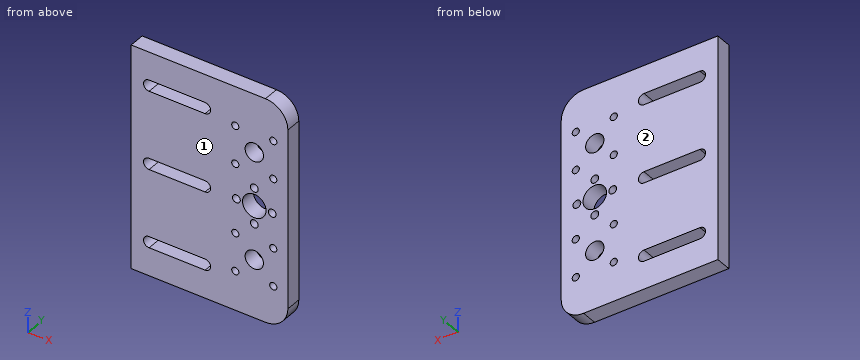
from build123d import *

# Parameters (mm, degrees)
SKETCH1_R           = 1.6
SKETCH1_R_2         = 4.1
SKETCH1_R_3         = 1.75
SKETCH1_R_4         = 5.25
BOSS_EXTRUDE1_DEPTH = 7
FILLET1_R           = 10


with BuildPart() as part:
    # Sketch1 → Boss-Extrude1 (new body)
    # profile 1 of 3: a face of its own
    with BuildSketch(Plane(origin=(0, 0, 0), x_dir=(1, 0, 0), z_dir=(0, 1, 0))):
        Polygon((0, 100), (0, 0), (56, 0), (70, 0), (70, 100), align=None)
        with BuildLine():
            Line((33, 12.5), (8, 12.5))
            ThreePointArc((8, 12.5), (5.5, 15), (8, 17.5))
            Line((8, 17.5), (33, 17.5))
            ThreePointArc((33, 17.5), (35.5, 15), (33, 12.5))
        make_face(mode=Mode.SUBTRACT)
        with Locations(Location((46.51, 17.51, 0), (0, 0, 270))):
            Circle(SKETCH1_R, mode=Mode.SUBTRACT)
        with Locations(Location((63.49, 17.51, 0), (0, 0, 270))):
            Circle(SKETCH1_R, mode=Mode.SUBTRACT)
        with Locations(Location((46.51, 34.49, 0), (0, 0, 270))):
            Circle(SKETCH1_R, mode=Mode.SUBTRACT)
        with Locations(Location((55, 26, 0), (0, 0, 270))):
            Circle(SKETCH1_R_2, mode=Mode.SUBTRACT)
        with Locations(Location((63.49, 34.49, 0), (0, 0, 270))):
            Circle(SKETCH1_R, mode=Mode.SUBTRACT)
        with Locations(Location((55, 42, 0), (0, 0, 270))):
            Circle(SKETCH1_R_3, mode=Mode.SUBTRACT)
        with BuildLine():
            ThreePointArc((8, 47.5), (5.5, 50), (8, 52.5))
            Line((8, 52.5), (33, 52.5))
            ThreePointArc((33, 52.5), (35.5, 50), (33, 47.5))
            Line((33, 47.5), (8, 47.5))
        make_face(mode=Mode.SUBTRACT)
        with BuildLine():
            ThreePointArc((8, 82.5), (5.5, 85), (8, 87.5))
            Line((8, 87.5), (33, 87.5))
            ThreePointArc((33, 87.5), (35.5, 85), (33, 82.5))
            Line((33, 82.5), (8, 82.5))
        make_face(mode=Mode.SUBTRACT)
        with Locations(Location((47, 50, 0), (0, 0, 270))):
            Circle(SKETCH1_R_3, mode=Mode.SUBTRACT)
        with Locations(Location((46.51, 65.51, 0), (0, 0, 270))):
            Circle(SKETCH1_R, mode=Mode.SUBTRACT)
        with Locations(Location((55, 50, 0), (0, 0, 270))):
            Circle(SKETCH1_R_4, mode=Mode.SUBTRACT)
        with Locations(Location((55, 58, 0), (0, 0, 270))):
            Circle(SKETCH1_R_3, mode=Mode.SUBTRACT)
        with Locations(Location((63, 50, 0), (0, 0, 270))):
            Circle(SKETCH1_R_3, mode=Mode.SUBTRACT)
        with Locations(Location((55, 74, 0), (0, 0, 270))):
            Circle(SKETCH1_R_2, mode=Mode.SUBTRACT)
        with Locations(Location((63.49, 65.51, 0), (0, 0, 270))):
            Circle(SKETCH1_R, mode=Mode.SUBTRACT)
        with Locations(Location((46.51, 82.49, 0), (0, 0, 270))):
            Circle(SKETCH1_R, mode=Mode.SUBTRACT)
        with Locations(Location((63.49, 82.49, 0), (0, 0, 270))):
            Circle(SKETCH1_R, mode=Mode.SUBTRACT)
    # profile 2 of 3: a face of its own
    with BuildSketch(Plane(origin=(0, 0, 0), x_dir=(1, 0, 0), z_dir=(0, 1, 0))):
        Polygon((0, 100), (0, 0), (56, 0), (70, 0), (70, 100), align=None)
        with BuildLine():
            Line((33, 12.5), (8, 12.5))
            ThreePointArc((8, 12.5), (5.5, 15), (8, 17.5))
            Line((8, 17.5), (33, 17.5))
            ThreePointArc((33, 17.5), (35.5, 15), (33, 12.5))
        make_face(mode=Mode.SUBTRACT)
        with Locations(Location((46.51, 17.51, 0), (0, 0, 270))):
            Circle(SKETCH1_R, mode=Mode.SUBTRACT)
        with Locations(Location((63.49, 17.51, 0), (0, 0, 270))):
            Circle(SKETCH1_R, mode=Mode.SUBTRACT)
        with Locations(Location((46.51, 34.49, 0), (0, 0, 270))):
            Circle(SKETCH1_R, mode=Mode.SUBTRACT)
        with Locations(Location((55, 26, 0), (0, 0, 270))):
            Circle(SKETCH1_R_2, mode=Mode.SUBTRACT)
        with Locations(Location((63.49, 34.49, 0), (0, 0, 270))):
            Circle(SKETCH1_R, mode=Mode.SUBTRACT)
        with Locations(Location((55, 42, 0), (0, 0, 270))):
            Circle(SKETCH1_R_3, mode=Mode.SUBTRACT)
        with BuildLine():
            ThreePointArc((8, 47.5), (5.5, 50), (8, 52.5))
            Line((8, 52.5), (33, 52.5))
            ThreePointArc((33, 52.5), (35.5, 50), (33, 47.5))
            Line((33, 47.5), (8, 47.5))
        make_face(mode=Mode.SUBTRACT)
        with BuildLine():
            ThreePointArc((8, 82.5), (5.5, 85), (8, 87.5))
            Line((8, 87.5), (33, 87.5))
            ThreePointArc((33, 87.5), (35.5, 85), (33, 82.5))
            Line((33, 82.5), (8, 82.5))
        make_face(mode=Mode.SUBTRACT)
        with Locations(Location((47, 50, 0), (0, 0, 270))):
            Circle(SKETCH1_R_3, mode=Mode.SUBTRACT)
        with Locations(Location((46.51, 65.51, 0), (0, 0, 270))):
            Circle(SKETCH1_R, mode=Mode.SUBTRACT)
        with Locations(Location((55, 50, 0), (0, 0, 270))):
            Circle(SKETCH1_R_4, mode=Mode.SUBTRACT)
        with Locations(Location((55, 58, 0), (0, 0, 270))):
            Circle(SKETCH1_R_3, mode=Mode.SUBTRACT)
        with Locations(Location((63, 50, 0), (0, 0, 270))):
            Circle(SKETCH1_R_3, mode=Mode.SUBTRACT)
        with Locations(Location((55, 74, 0), (0, 0, 270))):
            Circle(SKETCH1_R_2, mode=Mode.SUBTRACT)
        with Locations(Location((63.49, 65.51, 0), (0, 0, 270))):
            Circle(SKETCH1_R, mode=Mode.SUBTRACT)
        with Locations(Location((46.51, 82.49, 0), (0, 0, 270))):
            Circle(SKETCH1_R, mode=Mode.SUBTRACT)
        with Locations(Location((63.49, 82.49, 0), (0, 0, 270))):
            Circle(SKETCH1_R, mode=Mode.SUBTRACT)
    # profile 3 of 3: a face of its own
    with BuildSketch(Plane(origin=(0, 0, 0), x_dir=(1, 0, 0), z_dir=(0, 1, 0))):
        Polygon((0, 100), (0, 0), (56, 0), (70, 0), (70, 100), align=None)
        with BuildLine():
            Line((33, 12.5), (8, 12.5))
            ThreePointArc((8, 12.5), (5.5, 15), (8, 17.5))
            Line((8, 17.5), (33, 17.5))
            ThreePointArc((33, 17.5), (35.5, 15), (33, 12.5))
        make_face(mode=Mode.SUBTRACT)
        with Locations(Location((46.51, 17.51, 0), (0, 0, 270))):
            Circle(SKETCH1_R, mode=Mode.SUBTRACT)
        with Locations(Location((63.49, 17.51, 0), (0, 0, 270))):
            Circle(SKETCH1_R, mode=Mode.SUBTRACT)
        with Locations(Location((46.51, 34.49, 0), (0, 0, 270))):
            Circle(SKETCH1_R, mode=Mode.SUBTRACT)
        with Locations(Location((55, 26, 0), (0, 0, 270))):
            Circle(SKETCH1_R_2, mode=Mode.SUBTRACT)
        with Locations(Location((63.49, 34.49, 0), (0, 0, 270))):
            Circle(SKETCH1_R, mode=Mode.SUBTRACT)
        with Locations(Location((55, 42, 0), (0, 0, 270))):
            Circle(SKETCH1_R_3, mode=Mode.SUBTRACT)
        with BuildLine():
            ThreePointArc((8, 47.5), (5.5, 50), (8, 52.5))
            Line((8, 52.5), (33, 52.5))
            ThreePointArc((33, 52.5), (35.5, 50), (33, 47.5))
            Line((33, 47.5), (8, 47.5))
        make_face(mode=Mode.SUBTRACT)
        with BuildLine():
            ThreePointArc((8, 82.5), (5.5, 85), (8, 87.5))
            Line((8, 87.5), (33, 87.5))
            ThreePointArc((33, 87.5), (35.5, 85), (33, 82.5))
            Line((33, 82.5), (8, 82.5))
        make_face(mode=Mode.SUBTRACT)
        with Locations(Location((47, 50, 0), (0, 0, 270))):
            Circle(SKETCH1_R_3, mode=Mode.SUBTRACT)
        with Locations(Location((46.51, 65.51, 0), (0, 0, 270))):
            Circle(SKETCH1_R, mode=Mode.SUBTRACT)
        with Locations(Location((55, 50, 0), (0, 0, 270))):
            Circle(SKETCH1_R_4, mode=Mode.SUBTRACT)
        with Locations(Location((55, 58, 0), (0, 0, 270))):
            Circle(SKETCH1_R_3, mode=Mode.SUBTRACT)
        with Locations(Location((63, 50, 0), (0, 0, 270))):
            Circle(SKETCH1_R_3, mode=Mode.SUBTRACT)
        with Locations(Location((55, 74, 0), (0, 0, 270))):
            Circle(SKETCH1_R_2, mode=Mode.SUBTRACT)
        with Locations(Location((63.49, 65.51, 0), (0, 0, 270))):
            Circle(SKETCH1_R, mode=Mode.SUBTRACT)
        with Locations(Location((46.51, 82.49, 0), (0, 0, 270))):
            Circle(SKETCH1_R, mode=Mode.SUBTRACT)
        with Locations(Location((63.49, 82.49, 0), (0, 0, 270))):
            Circle(SKETCH1_R, mode=Mode.SUBTRACT)
    extrude(amount=BOSS_EXTRUDE1_DEPTH)

    # Fillet1
    fillet1_edges = [part.edges().sort_by_distance(p)[0] for p in [
        (70, 3.5, -100),
        (70, 3.5, 0),
    ]]
    fillet(fillet1_edges, radius=FILLET1_R)


solid = part.part
Read the model definition and answer for the solid it produces. Units are mm, in the model's axes. Face numbers are marked on the shaded views. Give positions to 0.01 mm unless a question says otherwise; leave off trailing zeros. Write each loop counter-clockwise with the first axis right and the second up, starting at its lowest first coordinate (ties: lowest second). Pieces come first, ordered by that corner, then holes. Notation, with made-up numbers: (82.25, 23.5) - (89.25, 23.5) arc R22 cw to (89.25, 57.5) - close; hole circle Ø1 at (15.5, -29.75). An arc over 180 degrees is marked (long way). Return JSON: item names as keys, results as strings.
Q1. A cutting plane is placed at A-A, the plane z = -58. Determine the outline of the cut face in (x, y).
Reply:
{"outline": "(0, 0) - (53.25, 0) - (53.25, 7) - (0, 7) - close; (56.75, 0) - (70, 0) - (70, 7) - (56.75, 7) - close"}
Q2. A cutting plane is placed at D-D, the plane y = 4.5. Count the separate pieces of the cut face and the enclosed holes in it, and give its area (3 significant figures).
Reply:
{"separate pieces": "1", "enclosed holes": "18", "area": "6,230 mm²"}
Q3. Given P1, Ø4.5, axis at x = 63, z = -50, coming from the -Y side; P2, Ø1.9, axis at x = 46.51, z = -82.49, coming from the -Y side, each flat-ended and moving along its own axis, determine where each tip first touches the part or whether it passes through.
Reply:
{"P1": "y = 0", "P2": "through"}
Q4. Consider line 1 along X through (y, z) = (4.25, -65.51); line 2 along Z through (x, y) = (25, 0.5); line 3 along X through (y, z) = (4.25, -26). Determine where each line is inside the solid, lowest interval first. Write a range as [from, to].
Reply:
{"line 1": "[0, 44.91], [48.11, 61.89], [65.09, 70]", "line 2": "[-100, -87.5], [-82.5, -52.5], [-47.5, -17.5], [-12.5, 0]", "line 3": "[0, 50.9], [59.1, 70]"}
Q5. A cutting plane is placed at C-C, the plane x = 27. Determine the outline of the cut face in (y, z).
Reply:
{"outline": "(0, -100) - (7, -100) - (7, -87.5) - (0, -87.5) - close; (0, -82.5) - (7, -82.5) - (7, -52.5) - (0, -52.5) - close; (0, -47.5) - (7, -47.5) - (7, -17.5) - (0, -17.5) - close; (0, -12.5) - (7, -12.5) - (7, 0) - (0, 0) - close"}
Q6. For a pull along Y with two mould halves and no side action, classify the marked faces 1 and 2 as released by +Y, released by -Y, zero draft, split by the parting line, or undercut.
Reply:
{"face 1": "released by -Y", "face 2": "released by +Y"}
Q7. A cutting plane is placed at B-B, the plane x = 55. Determine the outline of the cut face in (y, z), and give its area (3 significant figures).
Reply:
{"outline": "(0, -100) - (7, -100) - (7, -78.1) - (0, -78.1) - close; (0, -69.9) - (7, -69.9) - (7, -59.75) - (0, -59.75) - close; (0, -56.25) - (7, -56.25) - (7, -55.25) - (0, -55.25) - close; (0, -44.75) - (7, -44.75) - (7, -43.75) - (0, -43.75) - close; (0, -40.25) - (7, -40.25) - (7, -30.1) - (0, -30.1) - close; (0, -21.9) - (7, -21.9) - (7, 0) - (0, 0) - close", "area": "463 mm²"}
